Design review of the part built by this model. Coordinates are the model's own, in mm. A direction names the side the tool comes from. Coordinates: 2 decimals unless noted, no trailing zeros. Write each loop counter-clockwise with the first axis right and the second up, starting at its lowest first coordinate (ties: lowest second). Pieces come first, ordered by that corner, then holes. Notation, with made-up numbers: M 51,3 L 75,3 A14 ccw 75,30 Z; hole C 69,70.25 d3. An arc over 180 degrees is marked long. One line per question, with ' | ' between items.
from build123d import *

# Parameters (mm, degrees)
ESBO_O1_W                = 2.8
ESBO_O1_H                = 2.8
RESSALTO_EXTRUS_O1_DEPTH = 7


with BuildPart() as part:
    # Esboço1 → Ressalto-extrusão1 (new body)
    with BuildSketch(Plane.XY):
        with BuildLine():
            Line((13.312994231, 2.687005769), (12.025988463, 1.4))
            Line((12.025988463, 1.4), (-12.025988463, 1.4))
            Line((-12.025988463, 1.4), (-13.312994231, 2.687005769))
            ThreePointArc((-13.312994231, 2.687005769), (-16.56763954, 3.75736415), (-19.360846454, 1.773333333))
            ThreePointArc((-19.360846454, 1.773333333), (-19.618471303, 1.500555813), (-19.979949748, 1.4))
            Line((-19.979949748, 1.4), (-20.020050252, 1.4))
            ThreePointArc((-20.020050252, 1.4), (-20.381528697, 1.500555813), (-20.639153546, 1.773333333))
            ThreePointArc((-20.639153546, 1.773333333), (-27.8, 0), (-20.639153546, -1.773333333))
            ThreePointArc((-20.639153546, -1.773333333), (-20.381528697, -1.500555813), (-20.020050252, -1.4))
            Line((-20.020050252, -1.4), (-19.979949748, -1.4))
            ThreePointArc((-19.979949748, -1.4), (-19.618471303, -1.500555813), (-19.360846454, -1.773333333))
            ThreePointArc((-19.360846454, -1.773333333), (-16.56763954, -3.75736415), (-13.312994231, -2.687005769))
            Line((-13.312994231, -2.687005769), (-12.025988463, -1.4))
            Line((-12.025988463, -1.4), (12.025988463, -1.4))
            Line((12.025988463, -1.4), (13.312994231, -2.687005769))
            ThreePointArc((13.312994231, -2.687005769), (16.56763954, -3.75736415), (19.360846454, -1.773333333))
            ThreePointArc((19.360846454, -1.773333333), (19.618471303, -1.500555813), (19.979949748, -1.4))
            Line((19.979949748, -1.4), (20.020050252, -1.4))
            ThreePointArc((20.020050252, -1.4), (20.381528697, -1.500555813), (20.639153546, -1.773333333))
            ThreePointArc((20.639153546, -1.773333333), (27.8, 0), (20.639153546, 1.773333333))
            ThreePointArc((20.639153546, 1.773333333), (20.381528697, 1.500555813), (20.020050252, 1.4))
            Line((20.020050252, 1.4), (19.979949748, 1.4))
            ThreePointArc((19.979949748, 1.4), (19.618471303, 1.500555813), (19.360846454, 1.773333333))
            ThreePointArc((19.360846454, 1.773333333), (16.56763954, 3.75736415), (13.312994231, 2.687005769))
        make_face()
        with Locations((16, 0)):
            Rectangle(ESBO_O1_W, ESBO_O1_H, mode=Mode.SUBTRACT)
        with Locations((24, 0)):
            Rectangle(ESBO_O1_W, ESBO_O1_H, mode=Mode.SUBTRACT)
        with Locations((-24, 0)):
            Rectangle(ESBO_O1_W, ESBO_O1_H, mode=Mode.SUBTRACT)
        with Locations((-16, 0)):
            Rectangle(ESBO_O1_W, ESBO_O1_H, mode=Mode.SUBTRACT)
    extrude(amount=RESSALTO_EXTRUS_O1_DEPTH)


solid = part.part
1. Insertion check: pin 1 Ø3 at (x, z) = (-11, 4.5) entering from -Y; pin 2 Ø1.5 at (x, z) = (-8.5, 6) entering from -Y. Each pin has a flat end and moves straight along its axis. Give the tip position at first contact, or say it passes through.
Answer sheet:
pin 1: y = -1.87 | pin 2: y = -1.4
2. Draft analysis for pull direction Y (two halves, no side actions). For faces 1 (the face through (0, -1.4, 3)), 2 (the face through (-27.8, 0.1, 3.5)), 3 (the face through (17.4, 0, 3)), state which applies: pulls with the +Y half, pulls with the -Y half, needs draft (parallel to the pull), parting line crosses it, or undercut.
Answer sheet:
face 1: pulls with the -Y half | face 2: parting line crosses it | face 3: undercut
3. Take a section at B-B (y = 0). Write out the cut boundary in (x, z), then the cut area to 3 significant figures.
Answer sheet:
outline: M -27.8,0 L -25.4,0 L -25.4,7 L -27.8,7 Z; M -22.6,0 L -17.4,0 L -17.4,7 L -22.6,7 Z; M -14.6,0 L 14.6,0 L 14.6,7 L -14.6,7 Z; M 17.4,0 L 22.6,0 L 22.6,7 L 17.4,7 Z; M 25.4,0 L 27.8,0 L 27.8,7 L 25.4,7 Z | area: 311 mm^2
4. To check wall thickness, follow line 1 along X through (y, z) = (-1, 4); line 2 along X through (y, z) = (3, 0.75); line 3 along X through (y, z) = (1.75, 5.25). State the ranges of each line that lie inside material, in increasing order. Write a range as [from, to].
Answer sheet:
line 1: [-27.67, -25.4], [-22.6, -17.4], [-14.6, 14.6], [17.4, 22.6], [25.4, 27.67] | line 2: [-26.33, -21.67], [-18.33, -13.67], [13.67, 18.33], [21.67, 26.33] | line 3: [-27.37, -20.63], [-19.37, -12.38], [12.38, 19.37], [20.63, 27.37]
5. Take a section at A-A (x = -24). Write out the cut boundary in (y, z).
Answer sheet:
outline: M -3.8,0 L -1.4,0 L -1.4,7 L -3.8,7 Z; M 1.4,0 L 3.8,0 L 3.8,7 L 1.4,7 Z
6. Tool access review of faces 4 (the face through (12.66, -2.034, 3.451)), 5 (the face through (0, 0, 7)), 6 (the face through (-12.66, 2.034, 3.451)), 7 (the face through (24, -1.4, 3)): name each direction out of +Z, -Z, +X, -X, +Y, -Y from which nothing blocks a thin tool from reaching the whole face with its end or side.
Answer sheet:
face 4: +Z, -Z, -Y | face 5: +Z, +X, -X, +Y, -Y | face 6: +Z, -Z, +Y | face 7: +Z, -Z
7. Take a section at D-D (x = 2). Write out the cut boundary in (y, z).
Answer sheet:
outline: M -1.4,0 L 1.4,0 L 1.4,7 L -1.4,7 Z
8. Take a section at C-C (z = 1). Count the separate pieces of the cut face and the enclosed holes in it, then the cut area to 3 significant figures.
Answer sheet:
separate pieces: 1 | enclosed holes: 4 | area: 223 mm^2
